The model under review builds one solid part; all positions refer to its coordinate system, in mm. A direction names the side the tool comes from. Give positions to 0.01 mm unless a question says otherwise; leave off trailing zeros. Write each loop counter-clockwise with the first axis right and the second up, starting at its lowest first coordinate (ties: lowest second). Pieces come first, ordered by that corner, then holes. Notation, with made-up numbers: (-18, -19.75) -> (-12, -19.75) arc R8 ccw to (-12, -14.75) -> close; hole circle Ø7 at (77, 85.5). An arc over 180 degrees is marked (long way). Use CSV: the item, a comma, the result in double quotes.
```python
from build123d import *

# Parameters (mm, degrees)
ESBO_O1_R                = 13
RESSALTO_EXTRUS_O1_DEPTH = 20
ESBO_O4_R                = 3.3
CORTE_EXTRUS_O1_DEPTH    = 33.5
CHANFRO1_SIZE            = 3
CHANFRO3_SIZE            = 1
ESBO_O5_R                = 5.4
CORTE_EXTRUS_O2_DEPTH    = 1.5
ESBO_O6_R                = 2.75
CORTE_EXTRUS_O3_DEPTH    = 21


with BuildPart() as part:
    # Esboço1 → Ressalto-extrusão1 (new body)
    with BuildSketch(Plane.XY):
        Polygon((-30, -25), (-30, 7.5), (-17.5, 7.5), (-17.5, 18), (17.5, 18), (17.5, 7.5), (30, 7.5), (30, -25), align=None)
        Circle(ESBO_O1_R, mode=Mode.SUBTRACT)
    extrude(amount=RESSALTO_EXTRUS_O1_DEPTH)

    # Esboço4 → Corte-extrusão1 (cut, through all)
    with BuildSketch(Plane(origin=(0, 7.5, 0), x_dir=(1, 0, 0), z_dir=(0, 1, 0))):
        with Locations((-23, -10)):
            Circle(ESBO_O4_R)
        with Locations((23, -10)):
            Circle(ESBO_O4_R)
    extrude(amount=-CORTE_EXTRUS_O1_DEPTH, mode=Mode.SUBTRACT)

    # Chanfro1
    chanfro1_edges = [part.edges().sort_by_distance(p)[0] for p in [
        (-17.5, 18, 10),
        (17.5, 18, 10),
    ]]
    chamfer(chanfro1_edges, length=CHANFRO1_SIZE)

    # Chanfro3
    chanfro3_edges = [part.edges().sort_by_distance(p)[0] for p in [
        (23.75, 7.5, 20),
        (30, -8.75, 0),
        (0, -25, 0),
        (17.5, 11.25, 20),
        (-30, -25, 10),
        (-30, 7.5, 10),
        (30, 7.5, 10),
        (30, -25, 10),
        (-23.75, 7.5, 20),
        (-30, -8.75, 20),
        (0, 18, 0),
        (0, 18, 20),
        (-17.5, 11.25, 0),
        (-16, 16.5, 0),
        (0, -25, 20),
        (16, 16.5, 0),
        (-17.5, 11.25, 20),
        (-16, 16.5, 20),
        (16, 16.5, 20),
        (30, -8.75, 20),
        (-30, -8.75, 0),
        (-23.75, 7.5, 0),
        (17.5, 11.25, 0),
        (23.75, 7.5, 0),
    ]]
    chamfer(chanfro3_edges, length=CHANFRO3_SIZE)

    # Esboço5 → Corte-extrusão2 (cut)
    with BuildSketch(Plane(origin=(0, 7.5, 0), x_dir=(1, 0, 0), z_dir=(0, 1, 0))):
        with Locations((23, -10)):
            Circle(ESBO_O5_R)
        with Locations((-23, -10)):
            Circle(ESBO_O5_R)
    extrude(amount=-CORTE_EXTRUS_O2_DEPTH, mode=Mode.SUBTRACT)

    # Esboço6 → Corte-extrusão3 (cut, through all)
    with BuildSketch(Plane(origin=(0, 0, 0), x_dir=(-1, 0, 0), z_dir=(0, 0, -1))):
        with Locations((-23, 0)):
            Circle(ESBO_O6_R)
        with Locations((-23, -18)):
            Circle(ESBO_O6_R)
        with Locations((23, 0)):
            Circle(ESBO_O6_R)
        with Locations((23, -18)):
            Circle(ESBO_O6_R)
    extrude(amount=-CORTE_EXTRUS_O3_DEPTH, mode=Mode.SUBTRACT)


solid = part.part
```
Q1. To check wall thickness, follow probe 1 along Y at (x, z) = (-23, 5.25); probe 2 along X at (y, z) = (-14, 10); probe 3 along Z at (x, y) = (23, -9). State the ranges of each line that lie inside material, in increasing order.
Derived:
probe 1,"y = -25 to -20.75, -15.25 to -2.75, 2.75 to 6"
probe 2,"x = -30 to -26.3, -19.7 to 19.7, 26.3 to 30"
probe 3,"z = 0 to 6.7, 13.3 to 20"
Q2. Insertion check: pin 1 (7 mm diameter, centred on x = -23, y = -18, fed in from -Z); pin 2 (8.5 mm diameter, centred on x = -23, z = 10, fed in from +Y); pin 3 (6 mm diameter, centred on x = -24.5, z = 12.5, fed in from +Y); pin 4 (4 mm diameter, centred on y = 10, z = 8, fed in from +X). Each pin has a flat end and moves straight along its axis. Give the tip position at first contact, or say it passes through.
Derived:
pin 1,"stops at z = 0"
pin 2,"stops at y = 6"
pin 3,"stops at y = 7.5"
pin 4,"stops at x = 17.5"
Q3. The part is to be moulded in two halves that separate along X. For faces 1 (the cylindrical face through (-25.62, -17.17, 15.85)), 2 (the flat face through (15.62, 16.16, 19.51)), 3 (the flat face through (7, -12, 20)), 4 (the cylindrical face through (20.46, -1.05, 15.85)), say which applies: pulls with the +X half, pulls with the -X half, needs draft (parallel to the pull), parting line crosses it, or undercut.
Derived:
face 1,"undercut"
face 2,"pulls with the +X half"
face 3,"needs draft"
face 4,"undercut"
Q4. Consider section B-B (z = 10). State how many separate pieces and enclosed holes the cut face has, then the cut area to 3 significant figures.
Derived:
separate pieces,"3"
enclosed holes,"1"
area,"1,330 mm2"
Q5. Consider section A-A (x = 0). Write out the cut boundary in (y, z), then the cut area to 3 significant figures.
Derived:
outline,"(-25, 1) -> (-24, 0) -> (-13, 0) -> (-13, 20) -> (-24, 20) -> (-25, 19) -> close; (13, 0) -> (17, 0) -> (18, 1) -> (18, 19) -> (17, 20) -> (13, 20) -> close"
area,"338 mm2"
Q6. Consider section C-C (y = 0). Write out the cut boundary in (x, z).
Derived:
outline,"(-30, 1) -> (-29, 0) -> (-25.75, 0) -> (-25.75, 8.18) arc R3.3 cw to (-25.75, 11.82) -> (-25.75, 20) -> (-29, 20) -> (-30, 19) -> close; (-20.25, 0) -> (-13, 0) -> (-13, 20) -> (-20.25, 20) -> (-20.25, 11.82) arc R3.3 cw to (-20.25, 8.18) -> close; (13, 0) -> (20.25, 0) -> (20.25, 8.18) arc R3.3 cw to (20.25, 11.82) -> (20.25, 20) -> (13, 20) -> close; (25.75, 0) -> (29, 0) -> (30, 1) -> (30, 19) -> (29, 20) -> (25.75, 20) -> (25.75, 11.82) arc R3.3 cw to (25.75, 8.18) -> close"
Q7. Machinability: for faces 5 (the flat face through (-28.4, 7.5, 7.9)), 6 (the cylindrical face through (20.38, -17.17, 4.03)), 7 (the flat face through (17.5, 11, 10)), which of the approach directions +Z, -Z, +X, -X, +Y, -Y give a long, thin tool a straight path to every point of the face, cutting with its end or side? Answer none if there is none.
Derived:
face 5,"+Z, -Z, -X, +Y"
face 6,"+Z, -Z"
face 7,"+Z, -Z, +X, +Y"
